The listing builds one solid part. Answer for the finished solid, in the listing's coordinates (mm). A direction names the side the tool comes from. Give positions to 0.01 mm unless a question says otherwise; leave off trailing zeros. Loops run counter-clockwise (first coordinate to the right, second up) from the corner with the lowest first, then second, coordinate; pieces in that order, holes last. Notation, with made-up numbers: M 36,74.25 L 48,74.25 A19 ccw 48,82.25 Z; hole C 86,-3.5 d11. An arc over 180 degrees is marked long. One line per item, written item: value. Start each with the question number.
Q1. For faces 1 (the cylindrical face through (-0.661, 25.398, 14.113)), 2 (the flat face through (12.3, 0.5, 12)), determine the directions among +Z, -Z, +X, -X, +Y, -Y from which every point of the face is accessible in a straight line to the end or side of a thin tool.
Q2. A cutting plane is placed at A-A, the plane y = 0. Determine the outline of the cut face in (x, z) (3 decimals).
Q3. A cutting plane is placed at B-B, the plane x = 0. State how many separate pieces and enclosed holes the cut face has, and give its area (3 significant figures).
Q4. Flat-ended cylindrical pins translate along their axes: pin 1 (5 mm diameter, centred on x = 24.57, y = -14.19, fed in from +Z); pin 2 (3 mm diameter, centred on x = 0, y = 28.375, fed in from -Z). Find the tip coordinate at first contact, or state that the pin passes through.
Q5. Consider L1, parallel to Y at x = 0, z = 13.7 (3 decimals); L2, parallel to X at y = -15, z = 12.2; L3, parallel to X at y = -10.5, z = 14.1. Determine where each line is inside the solid, lowest interval first.
Q6. The mould has two halves that part along Y. Classify faces 3 (the cylindrical face through (14.289, 24.515, 12.986)), 4 (the cylindrical face through (28.375, -0.117, 12.986)), 5 (the cylindrical face through (14.09, -24.63, 12.99)): +Y half, -Y half, draft (parallel to the pull), parting line (faces both ways), or undercut.
from build123d import *

# Parameters (mm, degrees)
SKETCH020_R         = 11.5
PAD005_DEPTH        = 3
HOLE004_D           = 3.6
HOLE004_CBORE_D     = 6.1
HOLE004_CBORE_DEPTH = 1.8
FILLET001_R         = 1
CHAMFER008_SIZE     = 0.4


with BuildPart() as part:
    # Sketch020 → Pad005 (new body)
    with BuildSketch(Plane.XY):
        with BuildLine():
            ThreePointArc((3.675973, 29.952093), (0, 32.375), (-3.675973, 29.952093))
            ThreePointArc((-6.443598, 27.633687), (-4.783337, 28.462877), (-3.675973, 29.952093))
            ThreePointArc((-6.443598, 27.633687), (-14.1875, 24.573471), (-20.709676, 19.397163))
            ThreePointArc((-24.101286, 18.159532), (-22.257905, 18.37393), (-20.709676, 19.397163))
            ThreePointArc((-24.101286, 18.159532), (-28.037572, 16.1875), (-27.77726, 11.79256))
            ThreePointArc((-27.153274, 8.236524), (-27.041243, 10.088947), (-27.77726, 11.79256))
            ThreePointArc((-27.153274, 8.236524), (-28.375, 0), (-27.153274, -8.236524))
            ThreePointArc((-27.77726, -11.79256), (-27.041243, -10.088947), (-27.153274, -8.236524))
            ThreePointArc((-27.77726, -11.79256), (-28.037572, -16.1875), (-24.101286, -18.159532))
            ThreePointArc((-20.709676, -19.397163), (-22.257905, -18.37393), (-24.101286, -18.159532))
            ThreePointArc((-20.709676, -19.397163), (-14.1875, -24.573471), (-6.443598, -27.633687))
            ThreePointArc((-3.675973, -29.952093), (-4.783337, -28.462877), (-6.443598, -27.633687))
            ThreePointArc((-3.675973, -29.952093), (0, -32.375), (3.675973, -29.952093))
            ThreePointArc((6.443598, -27.633687), (4.783337, -28.462877), (3.675973, -29.952093))
            ThreePointArc((6.443598, -27.633687), (14.1875, -24.573471), (20.709676, -19.397163))
            ThreePointArc((24.101286, -18.159532), (22.257905, -18.37393), (20.709676, -19.397163))
            ThreePointArc((24.101286, -18.159532), (28.037572, -16.1875), (27.77726, -11.79256))
            ThreePointArc((27.153274, -8.236524), (27.041243, -10.088947), (27.77726, -11.79256))
            ThreePointArc((27.153274, -8.236524), (28.375, 0), (27.153274, 8.236524))
            ThreePointArc((27.77726, 11.79256), (27.041243, 10.088947), (27.153274, 8.236524))
            ThreePointArc((27.77726, 11.79256), (28.037572, 16.1875), (24.101286, 18.159532))
            ThreePointArc((20.709676, 19.397163), (22.257905, 18.37393), (24.101286, 18.159532))
            ThreePointArc((20.709676, 19.397163), (14.1875, 24.573471), (6.443598, 27.633687))
            ThreePointArc((3.675973, 29.952093), (4.783337, 28.462877), (6.443598, 27.633687))
        make_face()
        Circle(SKETCH020_R, mode=Mode.SUBTRACT)
    extrude(amount=PAD005_DEPTH)

    # Hole004 (through all)
    with Locations(Plane.XY.offset(3)):
        with Locations((0, 28.375), (24.573471, -14.1875), (-24.573471, -14.1875)):
            CounterBoreHole(HOLE004_D / 2, HOLE004_CBORE_D / 2, HOLE004_CBORE_DEPTH)

    # Fillet001
    fillet001_edges = [part.edges().sort_by_distance(p)[0] for p in [
        (-28.037572, -16.1875, 3),
    ]]
    fillet(fillet001_edges, radius=FILLET001_R)

    # Chamfer008
    chamfer008_edges = [part.edges().sort_by_distance(p)[0] for p in [
        (-11.5, 0, 3),
        (-11.5, 0, 0),
    ]]
    chamfer(chamfer008_edges, length=CHAMFER008_SIZE)


with BuildPart() as part_1:
    # Body007 placement: moved
    add(part.part.moved(Location((0, 0, 12))))


solid = part_1.part
Answer block:
1. face 1: +Z
1. face 2: -Z, +X, -X, +Y, -Y
2. outline: M -28.375,12 L -11.9,12 L -11.5,12.4 L -11.5,14.6 L -11.9,15 L -27.375,15 A1 ccw -28.375,14 Z; M 11.5,12.4 L 11.9,12 L 28.375,12 L 28.375,14 A1 ccw 27.375,15 L 11.9,15 L 11.5,14.6 Z
3. separate pieces: 3
3. enclosed holes: 0
3. area: 109 mm^2
4. pin 1: z = 13.2
4. pin 2: through
5. L1: -32.375 to -11.5, 11.5 to 25.325, 31.425 to 32.375
5. L2: -28.49 to -26.18, -22.97 to 22.97, 26.18 to 28.49
5. L3: -27.13 to -4.69, 4.69 to 27.13
6. face 3: +Y half
6. face 4: undercut
6. face 5: -Y half
